from build123d import *

# Parameters (mm, degrees)
ESQUISSE1_R             = 2
BOSS_EXTRU_1_DEPTH      = 14.5
ESQUISSE3_W             = 12
ESQUISSE3_H             = 6.5
ENL_V_MAT_EXTRU_1_DEPTH = 55.612269684
BOSS_EXTRU_2_DEPTH      = 25.5


with BuildPart() as part:
    # Esquisse1 → Boss.-Extru.1 (new body)
    with BuildSketch(Plane.XY):
        with BuildLine():
            Line((-25, -10), (-19.364230348, -10))
            ThreePointArc((-19.364230348, -10), (-18.046020427, -10.546020427), (-17.5, -11.864230348))
            Line((-17.5, -11.864230348), (-17.5, -13))
            ThreePointArc((-17.5, -13), (-14, -16.5), (-10.5, -13))
            Line((-10.5, -13), (-10.5, -11.864230348))
            ThreePointArc((-10.5, -11.864230348), (-9.953979573, -10.546020427), (-8.635769652, -10))
            Line((-8.635769652, -10), (9.635769652, -10))
            ThreePointArc((9.635769652, -10), (10.953979573, -10.546020427), (11.5, -11.864230348))
            Line((11.5, -11.864230348), (11.5, -13))
            ThreePointArc((11.5, -13), (15, -16.5), (18.5, -13))
            Line((18.5, -13), (18.5, -11.864230348))
            ThreePointArc((18.5, -11.864230348), (19.046020427, -10.546020427), (20.364230348, -10))
            Line((20.364230348, -10), (25, -10))
            Line((25, -10), (25, 10))
            Line((25, 10), (20.364230348, 10))
            ThreePointArc((20.364230348, 10), (19.046020427, 10.546020427), (18.5, 11.864230348))
            Line((18.5, 11.864230348), (18.5, 13))
            ThreePointArc((18.5, 13), (15, 16.5), (11.5, 13))
            Line((11.5, 13), (11.5, 11.864230348))
            ThreePointArc((11.5, 11.864230348), (10.953979573, 10.546020427), (9.635769652, 10))
            Line((9.635769652, 10), (-8.635769652, 10))
            ThreePointArc((-8.635769652, 10), (-9.953979573, 10.546020427), (-10.5, 11.864230348))
            Line((-10.5, 11.864230348), (-10.5, 13))
            ThreePointArc((-10.5, 13), (-14, 16.5), (-17.5, 13))
            Line((-17.5, 13), (-17.5, 11.864230348))
            ThreePointArc((-17.5, 11.864230348), (-18.046020427, 10.546020427), (-19.364230348, 10))
            Line((-19.364230348, 10), (-25, 10))
            Line((-25, 10), (-25, -10))
        make_face()
        with Locations(Location((-14, 13, 0), (0, 0, 180))):
            Circle(ESQUISSE1_R, mode=Mode.SUBTRACT)
        with Locations(Location((15, 13, 0), (0, 0, 180))):
            Circle(ESQUISSE1_R, mode=Mode.SUBTRACT)
        with Locations(Location((-14, -13, 0), (0, 0, 180))):
            Circle(ESQUISSE1_R, mode=Mode.SUBTRACT)
        with Locations(Location((15, -13, 0), (0, 0, 180))):
            Circle(ESQUISSE1_R, mode=Mode.SUBTRACT)
    extrude(amount=BOSS_EXTRU_1_DEPTH)

    # Esquisse3 → Enlèv. mat.-Extru.1 (cut, through all)
    with BuildSketch(Plane(origin=(25, 0, 0), x_dir=(0, 0, -1), z_dir=(1, 0, 0))):
        with Locations((-8.5, 13.25)):
            Rectangle(ESQUISSE3_W, ESQUISSE3_H)
        with Locations((-8.5, -13.25)):
            Rectangle(ESQUISSE3_W, ESQUISSE3_H)
    extrude(amount=-ENL_V_MAT_EXTRU_1_DEPTH, mode=Mode.SUBTRACT)

    # Esquisse4 → Boss.-Extru.2 (add)
    with BuildSketch(Plane.XY.offset(14.5)):
        with BuildLine():
            Line((-6.339745962, -5), (6.339745962, -5))
            ThreePointArc((6.339745962, -5), (25, 0), (6.339745962, 5))
            Line((6.339745962, 5), (-6.339745962, 5))
            ThreePointArc((-6.339745962, 5), (-25, 0), (-6.339745962, -5))
        make_face()
    extrude(amount=BOSS_EXTRU_2_DEPTH)


solid = part.part
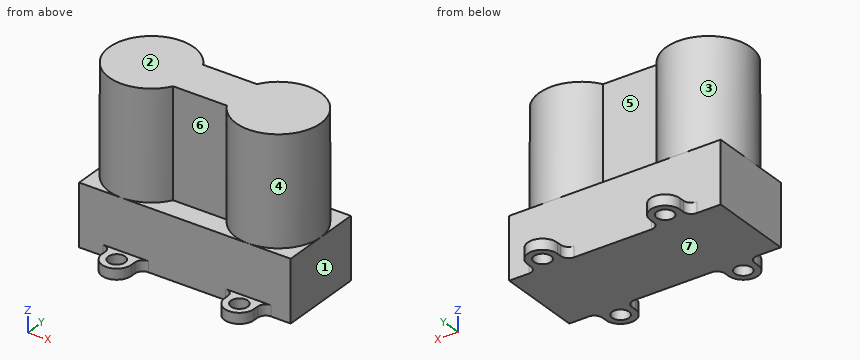
Build history of the part. All positions in model axes, mm. Face numbers are marked on the shaded views. A direction names the side the tool comes from. Round coordinates to 2 decimals unless told otherwise and drop trailing zeros. Write each loop counter-clockwise with the first axis right and the second up, starting at its lowest first coordinate (ties: lowest second). Pieces come first, ordered by that corner, then holes. Notation, with made-up numbers: M 70.25,67 L 88.25,67 A17 ccw 88.25,91 Z; hole C -15,-22.5 d5. An arc over 180 degrees is marked long. Answer in a Markdown table with one row per item.
1. Flat gauge pins, fed straight in: P1, Ø4, axis at x = 1, z = 29, coming from the +Y side; P2, Ø5, axis at y = -4.5, z = 35, coming from the -X side; P3, Ø2, axis at x = -12.5, y = -14, coming from the +Z side. Where does each tip first touch, or does it go through?
Geometry check:
| item | result |
|---|---|
| P1 | y = 5 |
| P2 | x = -24.8 |
| P3 | z = 2.5 |
2. Saw through at B-B (x = -14). List the corners of the cut face in (y, z).
Geometry check:
| item | result |
|---|---|
| outline | M -16.5,0 L -15,0 L -15,2.5 L -16.5,2.5 Z; M -11,0 L 11,0 L 11,2.5 L 10,2.5 L 10,14.5 L 9.95,14.5 L 9.95,40 L -9.95,40 L -9.95,14.5 L -10,14.5 L -10,2.5 L -11,2.5 Z; M 15,0 L 16.5,0 L 16.5,2.5 L 15,2.5 Z |
3. Saw through at C-C (y = -3.5). List the corners of the cut face in (x, z).
Geometry check:
| item | result |
|---|---|
| outline | M -25,0 L 25,0 L 25,14.5 L 24.37,14.5 L 24.37,40 L -24.37,40 L -24.37,14.5 L -25,14.5 Z |
4. Mould opens along X. For the marked faces 1, 2, 3 and 4 say: +X half, -X half, draft (parallel to the pull), parting line (faces both ways), or undercut.
Geometry check:
| item | result |
|---|---|
| face 1 | +X half |
| face 2 | draft |
| face 3 | undercut |
| face 4 | undercut |
5. Saw through at D-D (z = 22). List the corners of the cut face in (x, y).
Geometry check:
| item | result |
|---|---|
| outline | M -6.34,-5 L 6.34,-5 A10 ccw long 6.34,5 L -6.34,5 A10 ccw long Z |
6. Which spindle directions (+Z, -Z, +X, -X, +Y, -Y) get a long thin tool onto all of the face, cutting with end or side? Do the marked faces 5, 6 and 7. Say none if no direction does.
Geometry check:
| item | result |
|---|---|
| face 5 | +Z, +Y |
| face 6 | +Z, -Y |
| face 7 | -Z, +X, -X, +Y, -Y |
7. Probe L1, parallel to X at y = -13, z = 1; L2, parallel to Y at x = -14, z = 1.1; L3, parallel to Y at x = -2, z = 7. List the from-to ranges inside material, lowest first. Write a range as [from, to].
Geometry check:
| item | result |
|---|---|
| L1 | [-17.5, -16], [-12, -10.5], [11.5, 13], [17, 18.5] |
| L2 | [-16.5, -15], [-11, 11], [15, 16.5] |
| L3 | [-10, 10] |
8. Saw through at A-A (x = -7). List the corners of the cut face in (y, z).
Geometry check:
| item | result |
|---|---|
| outline | M -10,0 L 10,0 L 10,14.5 L 6,14.5 L 6,40 L -6,40 L -6,14.5 L -10,14.5 Z |
